Geometry check sheet. Reference: the model listing, model coordinates, mm. A direction names the side the tool comes from. Round coordinates to 2 decimals unless told otherwise and drop trailing zeros. Order: outer loops, then holes, each group sorted by start corner. A loop starts at its lowest first (then second) coordinate and runs counter-clockwise, first axis right, second up. Notation, with made-up numbers: (53, 54.5) - (95, 54.5) arc R29 cw to (95, 79.5) - close; hole circle Ø4 at (-38.5, 2). An arc over 180 degrees is marked (long way). Write each question's results on one line, items separated by ' | '.
```python
from build123d import *

# Parameters (mm, degrees)
ESQUISSE1_W             = 142
ESQUISSE1_H             = 74
BOSS_EXTRU_1_DEPTH      = 1
ESQUISSE2_W             = 142
ESQUISSE2_H             = 74
ESQUISSE2_W_2           = 140
ESQUISSE2_H_2           = 72
BOSS_EXTRU_2_DEPTH      = 32
ESQUISSE3_W             = 6
ESQUISSE3_H             = 6
BOSS_EXTRU_3_DEPTH      = 15
CHANFREIN1_SIZE         = 5
CHANFREIN1_SIZE2        = 13.737387097
CHANFREIN1_PART_2_SIZE  = 5
CHANFREIN1_PART_2_SIZE2 = 13.737387097
CHANFREIN1_PART_3_SIZE  = 5
CHANFREIN1_PART_3_SIZE2 = 13.737387097
CHANFREIN1_PART_4_SIZE  = 5
CHANFREIN1_PART_4_SIZE2 = 13.737387097
CHANFREIN1_PART_5_SIZE  = 5
CHANFREIN1_PART_5_SIZE2 = 13.737387097
CHANFREIN1_PART_6_SIZE  = 5
CHANFREIN1_PART_6_SIZE2 = 13.737387097
ESQUISSE4_R             = 1.1
ENL_V_MAT_EXTRU_1_DEPTH = 4
ESQUISSE5_R             = 2.5
ESQUISSE5_R_2           = 0.9
BOSS_EXTRU_4_DEPTH      = 4
ESQUISSE6_W             = 11.635872756
ESQUISSE6_H             = 12.977079273
ENL_V_MAT_EXTRU_2_DEPTH = 3


with BuildPart() as part:
    # Esquisse1 → Boss.-Extru.1 (new body)
    with BuildSketch(Plane.XY):
        with Locations((71, 37)):
            Rectangle(ESQUISSE1_W, ESQUISSE1_H)
    extrude(amount=BOSS_EXTRU_1_DEPTH)

    # Esquisse2 → Boss.-Extru.2 (add)
    with BuildSketch(Plane.XY.offset(1)):
        with Locations((71, 37)):
            Rectangle(ESQUISSE2_W, ESQUISSE2_H)
        with Locations((71, 37)):
            Rectangle(ESQUISSE2_W_2, ESQUISSE2_H_2, mode=Mode.SUBTRACT)
    extrude(amount=BOSS_EXTRU_2_DEPTH)

    # Esquisse3 → Boss.-Extru.3 (add)
    with BuildSketch(Plane.XY.offset(33)):
        with Locations((4, 70)):
            Rectangle(ESQUISSE3_W, ESQUISSE3_H)
        with Locations((138, 70)):
            Rectangle(ESQUISSE3_W, ESQUISSE3_H)
        with Locations((138, 4)):
            Rectangle(ESQUISSE3_W, ESQUISSE3_H)
        with Locations((4, 4)):
            Rectangle(ESQUISSE3_W, ESQUISSE3_H)
        with Locations((65, 4)):
            Rectangle(ESQUISSE3_W, ESQUISSE3_H)
        with Locations((65, 70)):
            Rectangle(ESQUISSE3_W, ESQUISSE3_H)
    extrude(amount=-BOSS_EXTRU_3_DEPTH)

    # Chanfrein1
    chanfrein1_edges = [part.edges().sort_by_distance(p)[0] for p in [
        (7, 70, 18),
        (4, 67, 18),
    ]]
    chanfrein1_side = [part.faces().sort_by_distance(p)[0] for p in [
        (4, 70, 18),
    ]]
    chamfer(chanfrein1_edges, length=CHANFREIN1_SIZE, length2=CHANFREIN1_SIZE2, reference=chanfrein1_side[0])

    # Chanfrein1 part 2
    chanfrein1_part_2_edges = [part.edges().sort_by_distance(p)[0] for p in [
        (138, 67, 18),
        (135, 70, 18),
    ]]
    chanfrein1_part_2_side = [part.faces().sort_by_distance(p)[0] for p in [
        (138, 70, 18),
    ]]
    chamfer(chanfrein1_part_2_edges, length=CHANFREIN1_PART_2_SIZE, length2=CHANFREIN1_PART_2_SIZE2, reference=chanfrein1_part_2_side[0])

    # Chanfrein1 part 3
    chanfrein1_part_3_edges = [part.edges().sort_by_distance(p)[0] for p in [
        (135, 4, 18),
        (138, 7, 18),
    ]]
    chanfrein1_part_3_side = [part.faces().sort_by_distance(p)[0] for p in [
        (138, 4, 18),
    ]]
    chamfer(chanfrein1_part_3_edges, length=CHANFREIN1_PART_3_SIZE, length2=CHANFREIN1_PART_3_SIZE2, reference=chanfrein1_part_3_side[0])

    # Chanfrein1 part 4
    chanfrein1_part_4_edges = [part.edges().sort_by_distance(p)[0] for p in [
        (4, 7, 18),
        (7, 4, 18),
    ]]
    chanfrein1_part_4_side = [part.faces().sort_by_distance(p)[0] for p in [
        (4, 4, 18),
    ]]
    chamfer(chanfrein1_part_4_edges, length=CHANFREIN1_PART_4_SIZE, length2=CHANFREIN1_PART_4_SIZE2, reference=chanfrein1_part_4_side[0])

    # Chanfrein1 part 5
    chanfrein1_part_5_edges = [part.edges().sort_by_distance(p)[0] for p in [
        (65, 7, 18),
    ]]
    chanfrein1_part_5_side = [part.faces().sort_by_distance(p)[0] for p in [
        (65, 4, 18),
    ]]
    chamfer(chanfrein1_part_5_edges, length=CHANFREIN1_PART_5_SIZE, length2=CHANFREIN1_PART_5_SIZE2, reference=chanfrein1_part_5_side[0])

    # Chanfrein1 part 6
    chanfrein1_part_6_edges = [part.edges().sort_by_distance(p)[0] for p in [
        (65, 67, 18),
    ]]
    chanfrein1_part_6_side = [part.faces().sort_by_distance(p)[0] for p in [
        (65, 70, 18),
    ]]
    chamfer(chanfrein1_part_6_edges, length=CHANFREIN1_PART_6_SIZE, length2=CHANFREIN1_PART_6_SIZE2, reference=chanfrein1_part_6_side[0])

    # Esquisse4 → Enlèv. mat.-Extru.1 (cut)
    with BuildSketch(Plane.XY.offset(33)):
        with Locations((4, 70)):
            Circle(ESQUISSE4_R)
        with Locations((65, 70)):
            Circle(ESQUISSE4_R)
        with Locations((138, 70)):
            Circle(ESQUISSE4_R)
        with Locations((138, 4)):
            Circle(ESQUISSE4_R)
        with Locations((65, 4)):
            Circle(ESQUISSE4_R)
        with Locations((4, 4)):
            Circle(ESQUISSE4_R)
    extrude(amount=-ENL_V_MAT_EXTRU_1_DEPTH, mode=Mode.SUBTRACT)

    # Esquisse5 → Boss.-Extru.4 (add)
    with BuildSketch(Plane.XY.offset(1)):
        with Locations((38, 62.5)):
            Circle(ESQUISSE5_R)
        with Locations((38, 62.5)):
            Circle(ESQUISSE5_R_2, mode=Mode.SUBTRACT)
        with Locations((68.48, 57.42)):
            Circle(ESQUISSE5_R)
        with Locations((68.48, 57.42)):
            Circle(ESQUISSE5_R_2, mode=Mode.SUBTRACT)
        with Locations((68.48, 29.48)):
            Circle(ESQUISSE5_R)
        with Locations((68.48, 29.48)):
            Circle(ESQUISSE5_R_2, mode=Mode.SUBTRACT)
        with Locations((44.336188826, 14.23343905)):
            Circle(ESQUISSE5_R)
        with Locations((44.336188826, 14.23343905)):
            Circle(ESQUISSE5_R_2, mode=Mode.SUBTRACT)
        with Locations((120.550955535, 62.5)):
            Circle(ESQUISSE5_R)
        with Locations((120.550955535, 62.5)):
            Circle(ESQUISSE5_R_2, mode=Mode.SUBTRACT)
        with Locations((119.28, 14.24)):
            Circle(ESQUISSE5_R)
        with Locations((119.28, 14.24)):
            Circle(ESQUISSE5_R_2, mode=Mode.SUBTRACT)
    extrude(amount=BOSS_EXTRU_4_DEPTH)

    # Esquisse6 → Enlèv. mat.-Extru.2 (cut)
    with BuildSketch(Plane(origin=(142, 0, 0), x_dir=(0, 0, -1), z_dir=(1, 0, 0))):
        with Locations((-12.35060992, 26.988539637)):
            Rectangle(ESQUISSE6_W, ESQUISSE6_H)
    extrude(amount=-ENL_V_MAT_EXTRU_2_DEPTH, mode=Mode.SUBTRACT)


solid = part.part
```
(1) Depth check by flat-ended pin: pin 1 Ø3 at (x, y) = (46.5, 8.5) entering from +Z; pin 2 Ø4 at (x, y) = (39, 62.5) entering from +Z. Enter the tip coordinate at first touch or a pass-through.
Answers follow:
pin 1: z = 1 | pin 2: z = 5
(2) Material ranges on line 1 (X direction, y = 29, z = 21.5); line 2 (Y direction, x = 65, z = 31); line 3 (Y direction, x = 89.5, z = 22), recorded low to high.
Answers follow:
line 1: 0 to 1, 141 to 142 | line 2: 0 to 2.9, 5.1 to 6.73, 67.27 to 68.9, 71.1 to 74 | line 3: 0 to 1, 73 to 74
(3) Section check C-C (x = 95). Record the cut outline in (y, z), then the cut area to 3 significant figures.
Answers follow:
outline: (0, 0) - (74, 0) - (74, 33) - (73, 33) - (73, 1) - (1, 1) - (1, 33) - (0, 33) - close | area: 138 mm²
(4) Access from +Z, -Z, +X, -X, +Y, -Y to the whole of each face (thin tool, end or side, straight path). Record for faces 4 (the face through (70, 74, 16)), 5 (the face through (1, 36, 17)), 6 (the face through (62, 71, 27)).
Answers follow:
face 4: +Z, -Z, +X, -X, +Y | face 5: none | face 6: +Z
(5) Section check B-B (z = 13). Record the cut outline in (x, y), then the cut area to 3 significant figures.
Answers follow:
outline: (0, 0) - (142, 0) - (142, 20.5) - (141, 20.5) - (141, 1) - (1, 1) - (1, 73) - (141, 73) - (141, 33.48) - (142, 33.48) - (142, 74) - (0, 74) - close | area: 415 mm²
(6) Draft check along Z on faces 1 (the face through (64.958, 4.535, 24.965)), 2 (the face through (45.4, 14.3, 5)), 3 (the face through (0, 36, 16)). Enter one of: released by +Z, released by -Z, zero draft, split by the parting line, or undercut.
Answers follow:
face 1: undercut | face 2: released by +Z | face 3: zero draft
(7) Section check A-A (y = 48). Record the cut outline in (x, z), then the cut area to 3 significant figures.
Answers follow:
outline: (0, 0) - (142, 0) - (142, 33) - (141, 33) - (141, 1) - (1, 1) - (1, 33) - (0, 33) - close | area: 206 mm²
